The listing builds one solid part. Answer for the finished solid, in the listing's coordinates (mm). A direction names the side the tool comes from. Give positions to 0.01 mm unless a question says otherwise; leave off trailing zeros. Order: outer loops, then holes, each group sorted by start corner. A loop starts at its lowest first (then second) coordinate and runs counter-clockwise, first axis right, second up.
```python
from build123d import *

# Parameters (mm, degrees)
F1_DEPTH = 30
F3_DEPTH = 15


with BuildPart() as f1:
    # F0 (on Front) → F1 (new body)
    with BuildSketch(Plane.XZ):
        Polygon((0, 30), (-15, 0), (15, 0), align=None)
    extrude(amount=F1_DEPTH)

    # F2 (on Right) → F3 (cut, symmetric)
    with BuildSketch(Plane.YZ):
        Polygon((0, 30), (-30, 30), (-30, 0), (-20, 10), (-20, 20), (-10, 20), align=None)
        Polygon((-20, 10), (-10, 20), (-20, 20), align=None)
        Polygon((-10, 10), (-10, 20), (-20, 10), align=None)
    extrude(amount=F3_DEPTH, both=True, mode=Mode.SUBTRACT)


solid = f1.part
```
1) Find section D-D (x = -1). Write down the section's boundary in (y, z), then the cut area to 3 significant figures.
Geometry says:
outline: (-30, 0) - (0, 0) - (0, 28) - (-2, 28) - (-10, 20) - (-10, 10) - (-20, 10) - close
area: 398 mm2
2) For a pull along Z with two mould halves and no side action, classify faces 1 (the flat face through (0, -15, 0)), 2 (the flat face through (9.27, -8.12, 11.46)), 3 (the flat face through (0, 0, 12)) as +Z half, -Z half, draft (parallel to the pull), parting line (faces both ways), or undercut.
Geometry says:
face 1: -Z half
face 2: +Z half
face 3: draft
3) A tool of negligible diameter and unlimited length cuts with its end or side. For faces 4 (the flat face through (-10.73, -8.12, 8.54)), 5 (the flat face through (0, -10, 14)), from which of +Z, -Z, +X, -X, +Y, -Y can it reach the whole face along a straight path? Write none if from no direction.
Geometry says:
face 4: +Z, -X, +Y, -Y
face 5: +Z, +X, -X, -Y
4) Find section C-C (y = -7). Write down the section's boundary in (x, z).
Geometry says:
outline: (-15, 0) - (15, 0) - (3.5, 23) - (-3.5, 23) - close
5) Find section A-A (x = -6.5). Write down the section's boundary in (y, z), then the cut area to 3 significant figures.
Geometry says:
outline: (-30, 0) - (0, 0) - (0, 17) - (-10, 17) - (-10, 10) - (-20, 10) - close
area: 320 mm2
6) Straight lines are drawn through the part: probe 1 along Z at (x, y) = (-8.75, -12); probe 2 along Y at (x, z) = (6, 15); probe 3 along Z at (x, y) = (4.75, -23). For each, find the intervals that lie inside material, in ascending order.
Geometry says:
probe 1: z = 0 to 10
probe 2: y = -10 to 0
probe 3: z = 0 to 7
7) Given P1, Ø4, axis at x = 6.5, z = 15.5, coming from the -Y side; P2, Ø4, axis at x = 7, y = -4, coming from the -Z side; P3, Ø11, axis at x = 1, y = -13.5, coming from the +Z side, each flat-ended and moving along its own axis, determine where each tip first touches the part or whether it passes through.
Geometry says:
P1: stops at y = -10
P2: stops at z = 0
P3: stops at z = 22
8) Find section B-B (z = 13). Write down the section's boundary in (x, y), then the cut area to 3 significant figures.
Geometry says:
outline: (-8.5, -10) - (8.5, -10) - (8.5, 0) - (-8.5, 0) - close
area: 170 mm2
